Answer from the drawing. Dimensions are ordinates in mm from the lowest x, y and z of the part. A direction names the side the tool comes from. Round coordinates to 2 decimals unless told otherwise and drop trailing zeros. Order: outer loops, then holes, each group sorted by start corner. A loop starts at its lowest first (then second) coordinate and runs counter-clockwise, first axis right, second up.
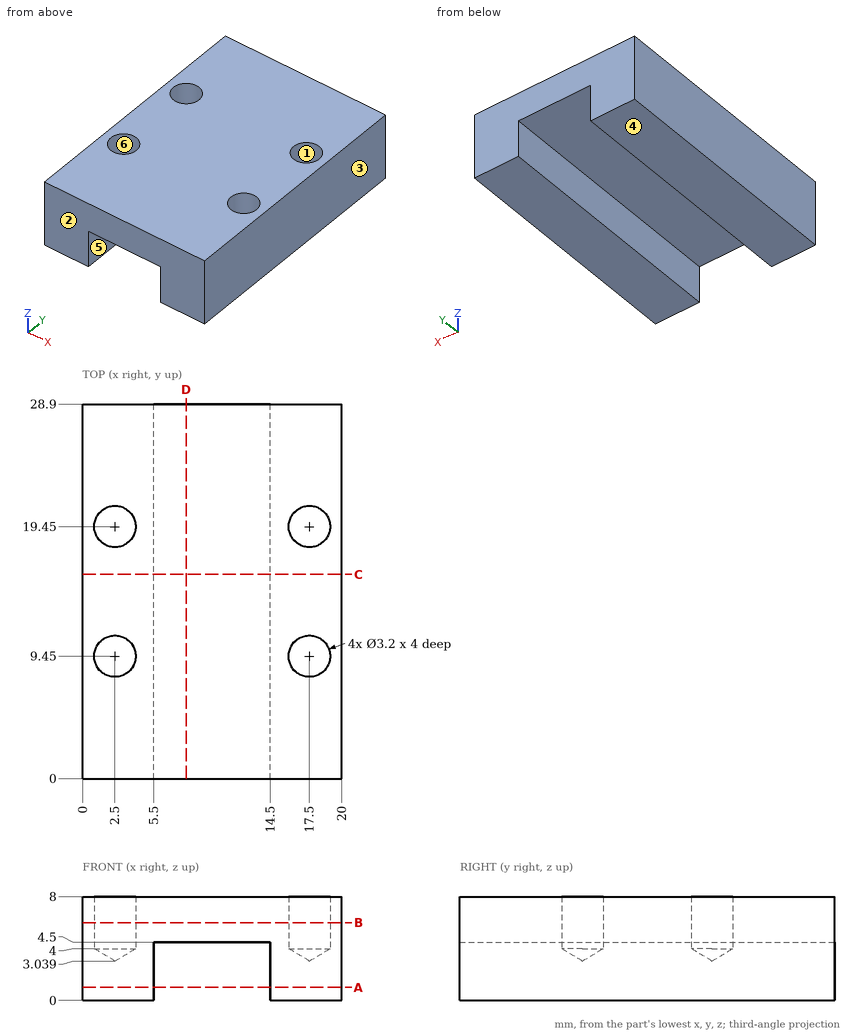
Q1. A cutting plane is placed at B-B, the plane z = 6. Give the vertices of the cut face in (x, y).
Outcome:
outline: (0, 0) - (20, 0) - (20, 28.9) - (0, 28.9) - close; hole circle Ø3.2 at (2.5, 9.45); hole circle Ø3.2 at (2.5, 19.45); hole circle Ø3.2 at (17.5, 9.45); hole circle Ø3.2 at (17.5, 19.45)
Q2. A cutting plane is placed at A-A, the plane z = 1. Give the vertices of the cut face in (x, y).
Outcome:
outline: (0, 0) - (5.5, 0) - (5.5, 28.9) - (0, 28.9) - close; (14.5, 0) - (20, 0) - (20, 28.9) - (14.5, 28.9) - close
Q3. For the marked faces 4, 5 and 6, determine the directions among +Z, -Z, +X, -X, +Y, -Y from which every point of the face is accessible in a straight line to the end or side of a thin tool.
Outcome:
face 4: -Z, +X, -X, +Y, -Y
face 5: -Z, +Y, -Y
face 6: +Z
Q4. Straight lines are drawn through the part: probe 1 along X at (y, z) = (9.45, 6.5); probe 2 along Y at (x, z) = (17.5, 6.7); probe 3 along X at (y, z) = (14.75, 1.75). For each, find the intervals that lie inside material, in ascending order.
Outcome:
probe 1: x = 0 to 0.9, 4.1 to 15.9, 19.1 to 20
probe 2: y = 0 to 7.85, 11.05 to 17.85, 21.05 to 28.9
probe 3: x = 0 to 5.5, 14.5 to 20
Q5. A cutting plane is placed at D-D, the plane x = 8. Give the vertices of the cut face in (y, z), plus the area to 3 significant figures.
Outcome:
outline: (0, 4.5) - (28.9, 4.5) - (28.9, 8) - (0, 8) - close
area: 101 mm2
Q6. A flat-ended cylindrical pin translates along its axis: pin 1 (2.5 mm diameter, centred on x = 9.5, y = 8.5, fed in from -Z). Find the tip coordinate at first contact, or state that the pin passes through.
Outcome:
pin 1: stops at z = 4.5
Q7. For a pull along Y with two mould halves and no side action, classify the marked faces 1, 2 and 3 as released by +Y, released by -Y, zero draft, split by the parting line, or undercut.
Outcome:
face 1: undercut
face 2: released by -Y
face 3: zero draft
Q8. A cutting plane is placed at C-C, the plane y = 15.75. Give the vertices of the cut face in (x, z), plus the area to 4 significant figures.
Outcome:
outline: (0, 0) - (5.5, 0) - (5.5, 4.5) - (14.5, 4.5) - (14.5, 0) - (20, 0) - (20, 8) - (0, 8) - close
area: 119.5 mm2
